from build123d import *

# Parameters (mm, degrees)
F0_W     = 1
F0_H     = 10
F1_DEPTH = 2
F0_W_2   = 1.5239776969
F0_W_3   = 1.4760223031
F0_W_4   = 2
F2_DEPTH = 1
F3_R     = 0.6
F4_R     = 1.1
F5_DEPTH = 50


with BuildPart() as f1:
    # F0 (on Front) → F1 (new body)
    with BuildSketch(Plane.XZ):
        with Locations((-46.041754216, 24.6294103354)):
            Rectangle(F0_W, F0_H)
    extrude(amount=-F1_DEPTH)



with BuildPart() as f1b:
    # F0 (on Front) → F1, piece 2 (new body)
    with BuildSketch(Plane.XZ):
        with Locations((-42.7797653675, 24.6294103354)):
            Rectangle(F0_W_2, F0_H)
    extrude(amount=-F1_DEPTH)


with BuildPart() as f1c:
    # F0 (on Front) → F1, piece 3 (new body)
    with BuildSketch(Plane.XZ):
        with Locations((-39.2797653675, 24.6294103354)):
            Rectangle(F0_W_3, F0_H)
    extrude(amount=-F1_DEPTH)


with BuildPart() as f1d:
    # F0 (on Front) → F1, piece 4 (new body)
    with BuildSketch(Plane.XZ):
        with Locations((-36.041754216, 24.6294103354)):
            Rectangle(F0_W, F0_H)
    extrude(amount=-F1_DEPTH)


with BuildPart() as f1_1:
    add(f1.part)

    add(f1b.part)  # F2 merges F1b

    add(f1c.part)  # F2 merges F1c

    add(f1d.part)  # F2 merges F1d
    # F0 (on Front) → F2 (join)
    with BuildSketch(Plane.XZ):
        with Locations((-41.0177765191, 24.6294103354)):
            Rectangle(F0_W_4, F0_H)
        with Locations((-39.2797653675, 24.6294103354)):
            Rectangle(F0_W_3, F0_H)
        with Locations((-46.041754216, 24.6294103354)):
            Rectangle(F0_W, F0_H)
        with Locations((-44.541754216, 24.6294103354)):
            Rectangle(F0_W_4, F0_H)
        with Locations((-36.041754216, 24.6294103354)):
            Rectangle(F0_W, F0_H)
        with Locations((-42.7797653675, 24.6294103354)):
            Rectangle(F0_W_2, F0_H)
        with Locations((-37.541754216, 24.6294103354)):
            Rectangle(F0_W_4, F0_H)
    extrude(amount=F2_DEPTH)

    # F3
    f3_edges = [f1_1.edges().sort_by_distance(p)[0] for p in [
        (-43.541754, 1, 29.62941),
        (-42.017777, 1, 29.62941),
        (-40.017777, 1, 19.62941),
        (-38.541754, 1, 19.62941),
        (-40.017777, 1, 29.62941),
        (-38.541754, 1, 29.62941),
        (-43.541754, 1, 19.62941),
        (-42.017777, 1, 19.62941),
        (-46.541754, 0.5, 19.62941),
        (-46.541754, 0.5, 29.62941),
        (-35.541754, 0.5, 29.62941),
        (-41.041754, -1, 29.62941),
        (-35.541754, -1, 24.62941),
        (-46.541754, -1, 24.62941),
        (-41.041754, -1, 19.62941),
        (-35.541754, 0.5, 19.62941),
    ]]
    fillet(f3_edges, radius=F3_R)

    # F4 (on Top) → F5 (cut)
    with BuildSketch(Plane.XY):
        with Locations((-37.5576429069, 1.0389162926)):
            Circle(F4_R)
        with Locations((-41.0279254586, 1.0422003123)):
            Circle(F4_R)
        with Locations((-44.5562924673, 1.0408099828)):
            Circle(F4_R)
    extrude(amount=F5_DEPTH, mode=Mode.SUBTRACT)


solid = f1_1.part
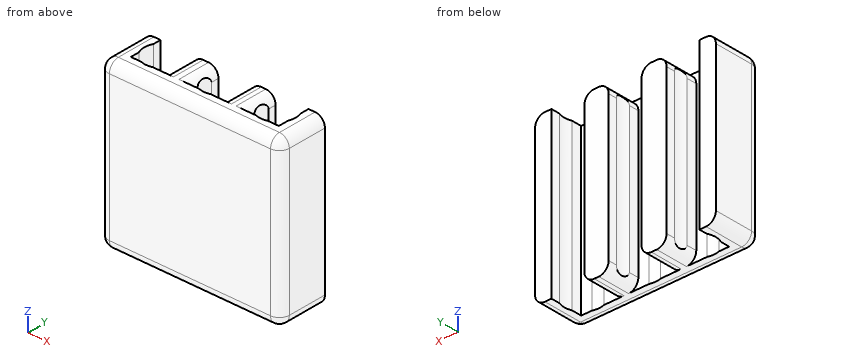
Verification items for the finished model (mm, model axes). Give positions to 0.01 mm unless a question says otherwise; leave off trailing zeros. Write each loop counter-clockwise with the first axis right and the second up, starting at its lowest first coordinate (ties: lowest second). Pieces come first, ordered by that corner, then holes. Notation, with made-up numbers: M 29.25,25 L 43.25,25 A11 ccw 43.25,29 Z; hole C -37,-11 d2. An arc over 180 degrees is marked long. Use CSV: the item, a comma, the result in double quotes.
1) Cross-section at D-D (y = 1). Enter the section's corners in (x, z), plus the area to 3 significant figures.
Final values:
outline,"M -46.54,20.23 A0.6 ccw -45.94,19.63 L -45.66,19.63 L -45.66,29.63 L -45.94,29.63 A0.6 ccw -46.54,29.03 Z; M -43.46,19.92 A0.6 ccw -42.94,19.63 L -42.62,19.63 A0.6 ccw -42.13,19.88 L -42.13,29.37 A0.6 ccw -42.62,29.63 L -42.94,29.63 A0.6 ccw -43.46,29.34 Z; M -39.93,19.91 A0.6 ccw -39.42,19.63 L -39.14,19.63 A0.6 ccw -38.66,19.88 L -38.66,29.38 A0.6 ccw -39.14,29.63 L -39.42,29.63 A0.6 ccw -39.93,29.34 Z; M -36.46,19.63 L -36.14,19.63 A0.6 ccw -35.54,20.23 L -35.54,29.03 A0.6 ccw -36.14,29.63 L -36.46,29.63 Z"
area,"43.4 mm²"
2) Material ranges on line 1 along X through (y, z) = (0.4, 23); line 2 along X through (y, z) = (1.2, 28); line 3 along Y through (x, z) = (-37, 26), recorded low to high.
Final values:
line 1,"-46.54 to -45.54, -43.54 to -42.02, -40.02 to -38.54, -36.54 to -35.54"
line 2,"-46.54 to -45.64, -43.47 to -42.12, -39.94 to -38.65, -36.47 to -35.54"
line 3,"-1 to 0"
3) Cross-section at A-A (y = 1.7). Enter the section's corners in (x, z).
Final values:
outline,"M -46.54,20.23 A0.6 ccw -45.94,19.63 L -45.54,19.63 L -45.54,29.63 L -45.94,29.63 A0.6 ccw -46.54,29.03 Z; M -43.54,20.23 A0.6 ccw -42.94,19.63 L -42.62,19.63 A0.6 ccw -42.02,20.23 L -42.02,29.03 A0.6 ccw -42.62,29.63 L -42.94,29.63 A0.6 ccw -43.54,29.03 Z; M -40.02,20.23 A0.6 ccw -39.42,19.63 L -39.14,19.63 A0.6 ccw -38.54,20.23 L -38.54,29.03 A0.6 ccw -39.14,29.63 L -39.42,29.63 A0.6 ccw -40.02,29.03 Z; M -36.54,19.63 L -36.14,19.63 A0.6 ccw -35.54,20.23 L -35.54,29.03 A0.6 ccw -36.14,29.63 L -36.54,29.63 Z"
4) Go/stop test with flat-tipped pins: pin 1 Ø1 at (x, z) = (-38.5, 24.5) entering from +Y; pin 2 Ø0.5 at (x, z) = (-37, 24) entering from +Y. Record where each tip stops, or that it passes through.
Final values:
pin 1,"y = 2"
pin 2,"y = 0"
5) Cross-section at B-B (x = -42.25). Enter the section's corners in (y, z), plus the area to 3 significant figures.
Final values:
outline,"M -1,20.23 A0.6 ccw -0.4,19.63 L 0,19.63 L 0,19.76 L 2,19.76 L 2,29.5 L 0,29.5 L 0,29.63 L -0.4,29.63 A0.6 ccw -1,29.03 Z"
area,"29.3 mm²"
6) Cross-section at C-C (y = -0.8). Enter the section's corners in (x, z).
Final values:
outline,"M -46.39,20.23 A0.45 ccw -45.94,19.78 L -36.14,19.78 A0.45 ccw -35.69,20.23 L -35.69,29.03 A0.45 ccw -36.14,29.48 L -45.94,29.48 A0.45 ccw -46.39,29.03 Z"
